Geometry check sheet. Reference: the model listing, model coordinates, mm. Face numbers are marked on the shaded views. A direction names the side the tool comes from. Coordinates: 2 decimals unless noted, no trailing zeros. Loops run counter-clockwise (first coordinate to the right, second up) from the corner with the lowest first, then second, coordinate; pieces in that order, holes last. Notation, with made-up numbers: (-17, -28.75) - (14, -28.75) arc R26 ccw to (14, 6.25) - close; hole circle Ø11 at (-36.75, 58). An arc over 180 degrees is marked (long way). Write each question's results on one line, items separated by ' | '. Start each with the question number.
(1) Sectioned sample at A-A (x = 10). Enter the section's corners in (y, z).
(2) Go/stop test with flat-tipped pins: pin 1 Ø2 at (x, z) = (49, 23.5) entering from +Y; pin 2 Ø12 at (y, z) = (8.5, 11.5) entering from +X; pin 3 Ø6 at (x, y) = (10, 55) entering from -Z; pin 4 Ø10.5 at (y, z) = (42, 21.7) entering from +X. Record where each tip stops, or that it passes through.
(3) Mould release check, pull along Y, two halves, no side actions. Record for the marked faces 3, 4 and 5: pulls with the +Y half, pulls with the -Y half, needs draft (parallel to the pull), parting line crosses it, or undercut.
(4) Sectioned sample at C-C (z = 20.7). Enter the section's corners in (x, y), plus the area to 3 significant figures.
(5) Sectioned sample at B-B (y = 55). Enter the section's corners in (x, z).
(6) Material ranges on probe 1 along Z at (x, y) = (9, 42); probe 2 along Z at (x, y) = (52, 3.25); probe 3 along X at (y, z) = (29.5, 8.5), recorded low to high.
(7) Access from +Z, -Z, +X, -X, +Y, -Y to the whole of each face (thin tool, end or side, straight path). Record for the marked faces 1 and 2.
(8) Sectioned sample at D-D (x = 36). Enter the section's corners in (y, z), plus the area to 3 significant figures.
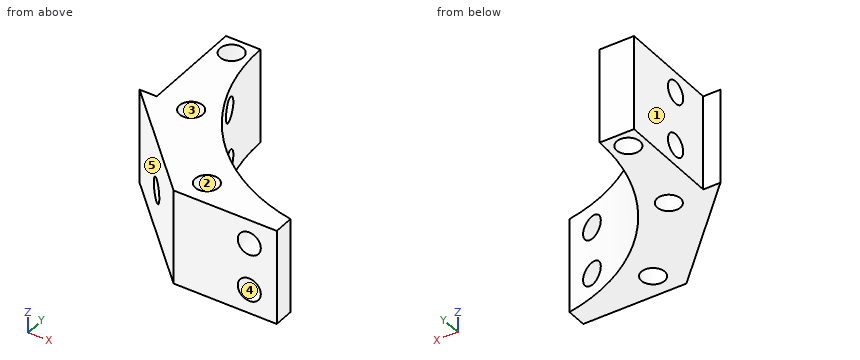
from build123d import *

# Parameters (mm, degrees)
SKETCH_1_W          = 30
SKETCH_1_H          = 30
SKETCH_1_W_2        = 25
EXTRUDE_1_DEPTH     = 27.7
SKETCH_3_R          = 55
CUT_EXTRUDE_1_DEPTH = 40
SKETCH_4_R          = 3.4
CUT_EXTRUDE_2_DEPTH = 90.259677346
SKETCH_5_R          = 3.3
CUT_EXTRUDE_3_DEPTH = 86.978427527
SKETCH_6_R          = 3.35
CUT_EXTRUDE_4_DEPTH = 90.259677512
EXTRUDE_2_DEPTH     = 50
SKETCH_8_R          = 3.4
CUT_EXTRUDE_5_DEPTH = 50
CUT_EXTRUDE_START   = -50
CUT_EXTRUDE_6_DEPTH = 50


with BuildPart() as part:
    # 草图1 → 凸台-拉伸1 (new body)
    with BuildSketch(Plane.XY):
        Polygon((0, 30), (30, 0), (30, 30), align=None)
        with Locations((45, 15)):
            Rectangle(SKETCH_1_W, SKETCH_1_H)
        with Locations((17.5, 45)):
            Rectangle(SKETCH_1_W_2, SKETCH_1_H)
    extrude(amount=EXTRUDE_1_DEPTH)

    # 草图3 → 切除-拉伸1 (cut)
    with BuildSketch(Plane.XY.offset(27.7)):
        with Locations((70, 60)):
            Circle(SKETCH_3_R)
    extrude(amount=-CUT_EXTRUDE_1_DEPTH, mode=Mode.SUBTRACT)

    # 草图4 → 切除-拉伸2 (cut, through all)
    with BuildSketch(Plane.XY.offset(27.7)):
        with Locations((35, 7)):
            Circle(SKETCH_4_R)
        with Locations((10, 55)):
            Circle(SKETCH_4_R)
        with Locations((15, 30)):
            Circle(SKETCH_4_R)
    extrude(amount=-CUT_EXTRUDE_2_DEPTH, mode=Mode.SUBTRACT)

    # 草图5 → 切除-拉伸3 (cut, through all)
    with BuildSketch(Plane.ZY.offset(-5)):
        with Locations(Location((6, 42, 0), (0, 0, 270))):
            Circle(SKETCH_5_R)
        with Locations(Location((21.7, 42, 0), (0, 0, 270))):
            Circle(SKETCH_5_R)
    extrude(amount=-CUT_EXTRUDE_3_DEPTH, mode=Mode.SUBTRACT)

    # 草图6 → 切除-拉伸4 (cut, through all)
    with BuildSketch(Plane.XZ):
        with Locations(Location((52, 20.7, 0), (0, 0, 270))):
            Circle(SKETCH_6_R)
        with Locations(Location((52, 7, 0), (0, 0, 270))):
            Circle(SKETCH_6_R)
    extrude(amount=-CUT_EXTRUDE_4_DEPTH, mode=Mode.SUBTRACT)

    # 草图7 → 凸台-拉伸2 (add)
    with BuildSketch(Plane(origin=(0, 0, 0), x_dir=(-1, 0, 0), z_dir=(0, 0, -1))):
        with BuildLine():
            Line((-5, 60), (-15, 60))
            ThreePointArc((-15, 60), (-27.721163687, 24.821881801), (-60, 5.916730868))
            Line((-60, 5.916730868), (-60, 0))
            Line((-60, 0), (-30, 0))
            Line((-30, 0), (0, 30))
            Line((0, 30), (-5, 30))
            Line((-5, 30), (-5, 60))
        make_face()
    extrude(amount=EXTRUDE_2_DEPTH)

    # 草图8 → 切除-拉伸5 (cut)
    with BuildSketch(Plane(origin=(15, 15, 0), x_dir=(0, 0, 1), z_dir=(-0.7071067811865477, -0.7071067811865475, 0))):
        with BuildLine():
            ThreePointArc((16.1, 0), (12.7, 3.4), (9.3, 0))
            Line((9.3, 0), (16.1, 0))
        make_face()
        with BuildLine():
            Line((16.1, 0), (9.3, 0))
            ThreePointArc((9.3, 0), (12.7, -3.4), (16.1, 0))
        make_face()
        with Locations(Location((-40, 10, 0), (0, 0, 270))):
            Circle(SKETCH_8_R)
        with Locations(Location((-20, 10, 0), (0, 0, 270))):
            Circle(SKETCH_8_R)
        with Locations(Location((-40, -10, 0), (0, 0, 270))):
            Circle(SKETCH_8_R)
        with Locations(Location((-20, -10, 0), (0, 0, 270))):
            Circle(SKETCH_8_R)
    extrude(amount=-CUT_EXTRUDE_5_DEPTH, mode=Mode.SUBTRACT)

    # 草图9 → 切除-拉伸6 (cut)
    with BuildSketch(Plane(origin=(0, 0, -50), x_dir=(-1, 0, 0), z_dir=(0, 0, -1)).offset(CUT_EXTRUDE_START)):
        with BuildLine():
            Line((-5, 30), (-5, 60))
            Line((-5, 60), (-15, 60))
            ThreePointArc((-15, 60), (-27.721163687, 24.821881801), (-60, 5.916730868))
            Line((-60, 5.916730868), (-60, 0))
            Line((-60, 0), (-30, 0))
            Line((-30, 0), (0, 30))
            Line((0, 30), (-5, 30))
        make_face()
    extrude(amount=CUT_EXTRUDE_6_DEPTH, mode=Mode.SUBTRACT)


solid = part.part
Outcome:
1) outline: (20, 0) - (51.6, 0) - (51.6, 27.7) - (20, 27.7) - close; (58.4, 0) - (60, 0) - (60, 27.7) - (58.4, 27.7) - close; hole circle Ø6.6 at (42, 6); hole circle Ø6.6 at (42, 21.7)
2) pin 1: stops at y = 9.59 | pin 2: stops at x = 60 | pin 3: passes through | pin 4: stops at x = 20.16
3) face 3: undercut | face 4: needs draft | face 5: pulls with the -Y half
4) outline: (0, 30) - (30, 0) - (48.65, 0) - (48.65, 9.31) arc R55 cw to (19.23, 38.86) - (5, 38.86) - (5, 30) - close; (5, 45.14) - (17.04, 45.14) arc R55 cw to (15, 60) - (5, 60) - close; (55.35, 0) - (60, 0) - (60, 5.92) arc R55 cw to (55.35, 6.99) - close; hole circle Ø6.8 at (10, 55); hole circle Ø6.8 at (15, 30); hole circle Ø6.8 at (35, 7) | area: 926 mm2
5) outline: (5, 0) - (6.6, 0) - (6.6, 27.7) - (5, 27.7) - close; (13.4, 0) - (15.23, 0) - (15.23, 27.7) - (13.4, 27.7) - close
6) probe 1: z = 0 to 2.7, 9.3 to 18.4, 25 to 27.7 | probe 2: z = 0 to 3.65, 10.35 to 17.35, 24.05 to 27.7 | probe 3: x = 0.5 to 11.64, 18.36 to 24.23
7) face 1: +Z, -Z, -X, +Y | face 2: +Z, -Z
8) outline: (0, 0) - (3.75, 0) - (3.75, 27.7) - (0, 27.7) - close; (10.25, 0) - (16.77, 0) - (16.77, 27.7) - (10.25, 27.7) - close | area: 284 mm2
